Part model, mm, in its own coordinate system. Face numbers are marked on the shaded views. A direction names the side the tool comes from. Round coordinates to 2 decimals unless told otherwise and drop trailing zeros. Order: outer loops, then holes, each group sorted by start corner. A loop starts at its lowest first (then second) coordinate and runs counter-clockwise, first axis right, second up. Notation, with made-up numbers: (12, -29.5) - (21, -29.5) arc R27 ccw to (21, 3.5) - close; hole circle Ø5 at (-37, -25). An arc over 180 degrees is marked (long way). Return JSON: item names as keys, results as strings. Group by question number.
Item 1: Probe probe 1 along Z at (x, y) = (-30, 5); probe 2 along Z at (x, y) = (-18, 69); probe 3 along X at (y, z) = (8, 54). List the from-to ranges inside material, lowest first.
Item 2: Saw through at B-B on y = 36. List the corners of the cut face in (x, z), and give its area (3 significant figures).
Item 3: Saw through at A-A on y = 66.5. List the corners of the cut face in (x, z), and give its area (3 significant figures).
Item 4: Saw through at C-C on y = 82.5. List the corners of the cut face in (x, z).
Item 5: Two-plate mould, pull along Z, no slides. Class the marked faces 1, 2, 3 and 4: released by +Z, released by -Z, zero draft, split by the parting line, or undercut.
Item 6: Drop flat-ended pins along their axis: pin 1 (5 mm diameter, centred on x = -65, y = -11.5, fed in from +Z); pin 2 (5 mm diameter, centred on x = -67, y = 1, fed in from -Z); pin 3 (4 mm diameter, centred on y = 28, z = 65.5, fed in from -X). Give the stop position or say it passes through.
Item 7: Tool access for the marked faces 5, 6 and 7: list every direction of +Z, -Z, +X, -X, +Y, -Y with a clear straight run to the whole face (end or side of a thin tool).
```python
from build123d import *

# Parameters (mm, degrees)
BOSS_EXTRUDE1_DEPTH      = 30
SKETCH2_W                = 40
SKETCH2_H                = 10
BOSS_EXTRUDE2_DEPTH      = 110
SKETCH3_W                = 40
SKETCH3_H                = 5
CUT_EXTRUDE1_DEPTH       = 50
SKETCH4_R                = 20
BOSS_EXTRUDE4_DEPTH      = 10
FILLET1_R                = 20
FILLET1_OF_MIRROR1_R     = 20
BOSS_EXTRUDE5_DEPTH      = 10
BOSS_EXTRUDE5_DEPTH_BACK = 30
SKETCH5_W                = 10
SKETCH5_H                = 20
BOSS_EXTRUDE6_DEPTH      = 20
BOSS_EXTRUDE6_DEPTH_BACK = 20
SKETCH6_R                = 5
FILLET2_R                = 2.5


with BuildPart() as part:
    # Sketch1 → Boss-Extrude1 (new body)
    with BuildSketch(Plane(origin=(0, 0, 0), x_dir=(1, 0, 0), z_dir=(0, 1, 0))):
        with BuildLine():
            Line((0, 65), (0, 60))
            ThreePointArc((0, 60), (-60, 0), (0, -60))
            Line((0, -60), (0, -65))
            ThreePointArc((0, -65), (-65, 0), (0, 65))
        make_face()
    extrude(amount=BOSS_EXTRUDE1_DEPTH)

    # Sketch2 → Boss-Extrude2 (add)
    with BuildSketch(Plane(origin=(0, 0, 0), x_dir=(1, 0, 0), z_dir=(0, 1, 0))):
        with Locations((0, 65)):
            Rectangle(SKETCH2_W, SKETCH2_H)
    boss_extrude2 = extrude(amount=BOSS_EXTRUDE2_DEPTH)

    # Sketch3 → Cut-Extrude1 (cut)
    with BuildSketch(Plane(origin=(0, 110, 0), x_dir=(1, 0, 0), z_dir=(0, 1, 0))):
        with Locations((0, 67.5)):
            Rectangle(SKETCH3_W, SKETCH3_H)
    cut_extrude1 = extrude(amount=-CUT_EXTRUDE1_DEPTH, mode=Mode.SUBTRACT)

    # Sketch4 → Boss-Extrude4 (add)
    with BuildSketch(Plane(origin=(0, 0, -65), x_dir=(-1, 0, 0), z_dir=(0, 0, -1))):
        with Locations((0, 90)):
            Circle(SKETCH4_R)
    boss_extrude4 = extrude(amount=BOSS_EXTRUDE4_DEPTH)

    # Fillet1
    fillet1_edges = [part.edges().sort_by_distance(p)[0] for p in [
        (20, 110, -62.5),
        (-20, 110, -62.5),
    ]]
    fillet(fillet1_edges, radius=FILLET1_R - 0.0001)  # a hair under: the kernel refuses the full size

    # Mirror1: Boss-Extrude2, Cut-Extrude1, Boss-Extrude4 across plane
    add(boss_extrude2.mirror(Plane.XY))
    add(cut_extrude1.mirror(Plane.XY), mode=Mode.SUBTRACT)
    add(boss_extrude4.mirror(Plane.XY))

    # Fillet1 of Mirror1
    fillet1_of_mirror1_edges = [part.edges().sort_by_distance(p)[0] for p in [
        (20, 110, 62.5),
        (-20, 110, 62.5),
    ]]
    fillet(fillet1_of_mirror1_edges, radius=FILLET1_OF_MIRROR1_R - 0.0001)  # a hair under: the kernel refuses the full size

    # Sketch5 → Boss-Extrude5 (add, two sides: drawn at the far end of the back side and taken through both)
    with BuildSketch(Plane.XZ.offset(-BOSS_EXTRUDE5_DEPTH_BACK)):
        with Locations((-65, 0)):
            Rectangle(SKETCH5_W, SKETCH5_H)
    extrude(amount=BOSS_EXTRUDE5_DEPTH + BOSS_EXTRUDE5_DEPTH_BACK)

    # Sketch6 → Boss-Extrude6 (add, two sides: drawn at the far end of the back side and taken through both)
    with BuildSketch(Plane.XY.offset(-BOSS_EXTRUDE6_DEPTH_BACK)):
        with Locations((-65, -10)):
            Circle(SKETCH6_R)
    extrude(amount=BOSS_EXTRUDE6_DEPTH + BOSS_EXTRUDE6_DEPTH_BACK)

    # Fillet2
    fillet2_edges = [part.edges().sort_by_distance(p)[0] for p in [
        (-20, 60.00005, 60),
        (20, 45.00005, 60),
        (0, 110, 60),
        (14.142164913, 104.142164913, 60),
        (-14.142164913, 104.142164913, 60),
    ]]
    fillet(fillet2_edges, radius=FILLET2_R)
    fillet2_2_edges = [part.edges().sort_by_distance(p)[0] for p in [
        (-60, 30, 0),
    ]]
    fillet(fillet2_2_edges, radius=FILLET2_R - 0.0001)  # a hair under: the kernel refuses the full size
    fillet2_3_edges = [part.edges().sort_by_distance(p)[0] for p in [
        (-20, 60.00005, -60),
        (-14.142164913, 104.142164913, -60),
        (0, 110, -60),
        (14.142164913, 104.142164913, -60),
        (20, 45.00005, -60),
    ]]
    fillet(fillet2_3_edges, radius=FILLET2_R)


solid = part.part
```
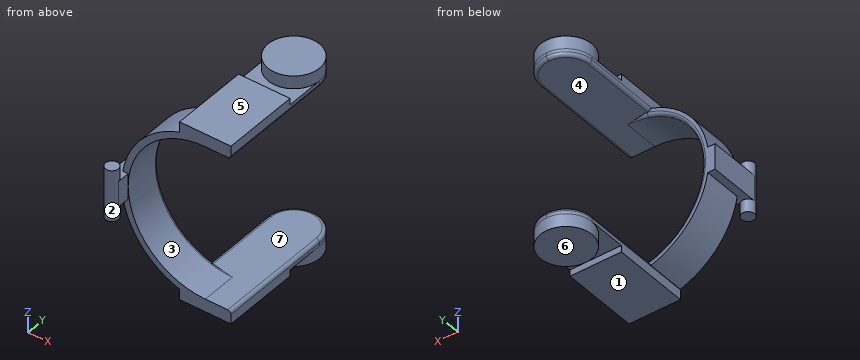
Filled in:
{
 "1": {"probe 1": "z = -57.66 to -51.96, 51.96 to 57.66", "probe 2": "z = -65 to -60.05, 60.05 to 65", "probe 3": "x = -36.18 to -26.15"},
 "2": {"outline": "(-20, -70) - (20, -70) - (20, -62.5) arc R2.5 ccw to (17.5, -60) - (-17.5, -60) arc R2.5 ccw to (-20, -62.5) - close; (-20, 62.5) arc R2.5 ccw to (-17.5, 60) - (17.5, 60) arc R2.5 ccw to (20, 62.5) - (20, 70) - (-20, 70) - close", "area": "795 mm^2"},
 "3": {"outline": "(-20, -65) - (20, -65) - (20, -62.5) arc R2.5 ccw to (17.5, -60) - (-17.5, -60) arc R2.5 ccw to (-20, -62.5) - close; (-20, 62.5) arc R2.5 ccw to (-17.5, 60) - (17.5, 60) arc R2.5 ccw to (20, 62.5) - (20, 65) - (-20, 65) - close", "area": "395 mm^2"},
 "4": {"outline": "(-20, -65) - (-18.54, -65) - (-18.54, -75) - (18.54, -75) - (18.54, -65) - (20, -65) - (20, -62.5) arc R2.5 ccw to (17.5, -60) - (-17.5, -60) arc R2.5 ccw to (-20, -62.5) - close; (-20, 62.5) arc R2.5 ccw to (-17.5, 60) - (17.5, 60) arc R2.5 ccw to (20, 62.5) - (20, 65) - (18.54, 65) - (18.54, 75) - (-18.54, 75) - (-18.54, 65) - (-20, 65) - close"},
 "5": {"face 1": "released by -Z", "face 2": "zero draft", "face 3": "undercut", "face 4": "undercut"},
 "6": {"pin 1": "stops at z = 20", "pin 2": "stops at z = -10", "pin 3": "stops at x = -20"},
 "7": {"face 5": "+Z, +X, -X, -Y", "face 6": "-Z, +X, -X, +Y, -Y", "face 7": "+X, +Y"}
}
